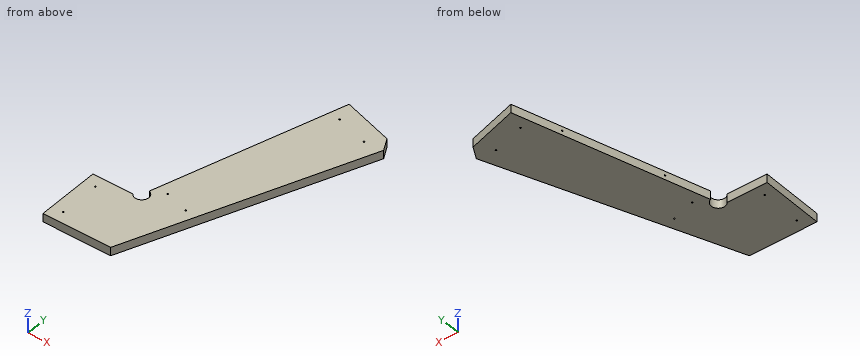
from build123d import *

# Parameters (mm, degrees)
BOSS_EXTRUDE1_DEPTH = 19.05
HOLE2_D             = 3.175
HOLE2_DEPTH         = 31.75
HOLE2_CSINK_D       = 10.16
HOLE2_CSINK_ANGLE   = 82
HOLE2_TIP           = 0.953866233
HOLE3_D             = 3.175
HOLE3_DEPTH         = 38.1
HOLE3_CSINK_D       = 10.16
HOLE3_CSINK_ANGLE   = 82
HOLE3_TIP           = 0.953866233


with BuildPart() as part:
    # Sketch1 → Boss-Extrude1 (new body)
    with BuildSketch(Plane.XY):
        with BuildLine():
            Line((-45.645654956, -462.283590669), (-42.196851456, -603.529354269))
            Line((-42.196851456, -603.529354269), (110.157739028, -599.809306096))
            Line((110.157739028, -599.809306096), (304.502022379, -82.799914861))
            Line((304.502022379, -82.799914861), (288.249001778, -54.142860136))
            Line((288.249001778, -54.142860136), (175.093421906, -22.889613201))
            Line((175.093421906, -22.889613201), (61.177817241, -435.332721236))
            ThreePointArc((61.177817241, -435.332721236), (69.660650717, -459.60790015), (43.950640658, -460.09591431))
            Line((43.950640658, -460.09591431), (-45.645654956, -462.283590669))
        make_face()
    extrude(amount=BOSS_EXTRUDE1_DEPTH)

    # Hole2
    with Locations(Plane(origin=(162.245907498, -21.702082459, 165.474999994), x_dir=(0, 0, -1), z_dir=(-0.963909776, 0.266229118, 0))):
        with Locations((-155.949999994, 107.734820482), (155.949999994, 107.734820482), (155.949999994, 327.755881328), (174.999999994, 85.732714397), (174.999999994, 349.757987412), (-174.999999994, 349.757987412), (-174.999999994, 85.732714397), (-155.949999994, 327.755881328)):
            CounterSinkHole(HOLE2_D / 2, HOLE2_CSINK_D / 2, depth=HOLE2_DEPTH, counter_sink_angle=HOLE2_CSINK_ANGLE)
            with Locations((0, 0, -(HOLE2_DEPTH + HOLE2_TIP / 2))):  # 118° drill point
                Cone(0, HOLE2_D / 2, HOLE2_TIP, mode=Mode.SUBTRACT)

    # Hole3
    with Locations(Plane(origin=(311.92831292, -63.043933951, -19.05), x_dir=(-0.351862635, -0.936051647, 0), z_dir=(0, 0, -1))):
        with Locations((46.221112845, 113.488854888), (39.39759596, 37.945520226), (412.28786892, 80.423559293), (407.308516105, 25.297013484), (513.561319184, 161.164706775), (597.46020397, 127.267357003), (610.543339245, 159.649253123), (694.322923815, 367.011001477), (526.644454459, 193.546602895), (610.424039029, 400.908351249)):
            CounterSinkHole(HOLE3_D / 2, HOLE3_CSINK_D / 2, depth=HOLE3_DEPTH, counter_sink_angle=HOLE3_CSINK_ANGLE)
            with Locations((0, 0, -(HOLE3_DEPTH + HOLE3_TIP / 2))):  # 118° drill point
                Cone(0, HOLE3_D / 2, HOLE3_TIP, mode=Mode.SUBTRACT)


solid = part.part
Could you check a few things on this model? Use its own coordinates, in mm. Round coordinates to 2 decimals unless told otherwise and drop trailing zeros. Order: outer loops, then holes, each group sorted by start corner. A loop starts at its lowest first (then second) coordinate and runs counter-clockwise, first axis right, second up. Notation, with made-up numbers: M -16,20.5 L 35,20.5 A37 ccw 35,56.5 Z; hole C 83.5,33.25 d11. An arc over 180 degrees is marked long. One line per item, written item: value.
(1) I need wall thicknesses on line 1 along Y through (x, z) = (-1, 11.5); line 2 along X through (y, z) = (-321.5, 6); line 3 along X through (y, z) = (-84, 2). Which ranges of each line are inside material? Lowest first, please. Write a range as from..to.
Ans:
line 1: y = -602.52..-461.19
line 2: x = 92.62..214.77
line 3: x = 158.21..304.05
(2) Imagine slicing it at A-A (y = -330). Write out the boundary of the cut face in (x, z).
Ans:
outline: M 90.27,0 L 211.58,0 L 211.58,19.05 L 90.27,19.05 Z
(3) I'm going to push flat-ended pins straight in: P1, Ø10, axis at x = 188, y = -139.5, coming from the -Z side; P2, Ø4, axis at y = -269, z = 5, coming from the -X side; P3, Ø10, axis at x = -9.5, z = 12.5, coming from the +Y side; P4, Ø4, axis at x = 214, z = 9.5, coming from the +Y side. Where does each tip first touch, or does it pass through?
Ans:
P1: stops at z = 0
P2: stops at x = 106.57
P3: stops at y = -461.28
P4: stops at y = -33.08
(4) Imagine slicing it at B-B (x = 215). Write out the boundary of the cut face in (y, z), and give its area (3 significant figures).
Ans:
outline: M -320.9,0 L -33.91,0 L -33.91,19.05 L -320.9,19.05 Z
area: 5,470 mm^2
